from build123d import *

# Parameters (mm, degrees)
BOSS_EXTRUDE1_DEPTH = 10
SKETCH2_W           = 40
SKETCH2_H           = 10
SKETCH2_R           = 1.5
BOSS_EXTRUDE2_DEPTH = 2
FILLET1_R           = 1
SKETCH3_R           = 1.6
CUT_EXTRUDE1_DEPTH  = 35.583232932


with BuildPart() as part:
    # Sketch1 → Boss-Extrude1 (new body)
    with BuildSketch(Plane.XY):
        Polygon((-10, 10), (-10, -10), (-10, -14), (-8, -14), (-8, -8), (-8, 8), (8, 8), (8, -8), (8, -14), (10, -14), (10, -10), (10, 10), align=None)
    extrude(amount=BOSS_EXTRUDE1_DEPTH)

    # Sketch2 → Boss-Extrude2 (add)
    with BuildSketch(Plane(origin=(0, 10, 0), x_dir=(1, 0, 0), z_dir=(0, 1, 0))):
        with Locations((0, -5)):
            Rectangle(SKETCH2_W, SKETCH2_H)
        with Locations(Location((-15, -5, 0), (0, 0, 270))):
            Circle(SKETCH2_R, mode=Mode.SUBTRACT)
        with Locations(Location((15, -5, 0), (0, 0, 90))):
            Circle(SKETCH2_R, mode=Mode.SUBTRACT)
    extrude(amount=BOSS_EXTRUDE2_DEPTH)

    # Fillet1
    fillet1_edges = [part.edges().sort_by_distance(p)[0] for p in [
        (-10, 10, 5),
        (10, 10, 5),
    ]]
    fillet(fillet1_edges, radius=FILLET1_R)

    # Sketch3 → Cut-Extrude1 (cut, through all)
    with BuildSketch(Plane(origin=(10, 0, 0), x_dir=(0, 0, -1), z_dir=(1, 0, 0))):
        with Locations((-5, -9.930512369)):
            Circle(SKETCH3_R)
    extrude(amount=-CUT_EXTRUDE1_DEPTH, mode=Mode.SUBTRACT)


solid = part.part
Geometry: final body of the model. Coordinates: model frame, mm. A direction names the side the tool comes from. Give positions to 0.01 mm unless a question says otherwise; leave off trailing zeros. Order: outer loops, then holes, each group sorted by start corner. A loop starts at its lowest first (then second) coordinate and runs counter-clockwise, first axis right, second up. Notation, with made-up numbers: (57, 58.5) -> (112, 58.5) arc R19 cw to (112, 90.5) -> close; hole circle Ø3 at (88, -6.5). An arc over 180 degrees is marked (long way). Answer as a JSON object with one key per item and string values.
Q1. Section D-D (z = 4.5). State how many separate pieces and enclosed holes the cut face has, plus the area to 3 significant figures.
Entries:
{"separate pieces": "5", "enclosed holes": "0", "area": "185 mm^2"}
Q2. Section B-B (x = -15). Output: boundary loops of the cut face in (y, z).
Entries:
{"outline": "(10, 0) -> (12, 0) -> (12, 3.5) -> (10, 3.5) -> close; (10, 6.5) -> (12, 6.5) -> (12, 10) -> (10, 10) -> close"}
Q3. Material intervals for probe 1 along X at (y, z) = (11.5, 5); probe 2 along X at (y, z) = (-7.75, 9.5); probe 3 along Z at (x, y) = (15, 11.3), sorted ascending.
Entries:
{"probe 1": "x = -20 to -16.5, -13.5 to 13.5, 16.5 to 20", "probe 2": "x = -10 to -8, 8 to 10", "probe 3": "z = 0 to 3.5, 6.5 to 10"}
Q4. Section A-A (y = -6.5). Output: boundary loops of the cut face in (x, z), plus the area to 3 significant figures.
Entries:
{"outline": "(-10, 0) -> (-8, 0) -> (-8, 10) -> (-10, 10) -> close; (8, 0) -> (10, 0) -> (10, 10) -> (8, 10) -> close", "area": "40.0 mm^2"}
Q5. Access query for faces 5 (the flat face through (0, 9, 10)), 6 (the flat face through (16.4, 10, 3.8)), 7 (the flat face through (-8, -3, 5)), 8 (the flat face through (-17, 10, 5)). Directions: +Z, -Z, +X, -X, +Y, -Y. A direction counts if a zero-diameter tool reaches every point of the face in a straight line with its end or side. Return the directions, or none.
Entries:
{"face 5": "+Z, +X, -X, +Y, -Y", "face 6": "+Z, -Z, +X, -Y", "face 7": "+Z, -Z, -Y", "face 8": "+Z, -Z, -X, -Y"}
Q6. Draft query along X for faces 1 (the flat face through (8, -3, 5)), 2 (the flat face through (10, -3, 5)), 3 (the cylindrical face through (14.93, 10.99, 6.5)), 4 (the cylindrical face through (-10.301, 9.715, 5.07)). Return one class per face: released by +X, released by -X, zero draft, split by the parting line, or undercut.
Entries:
{"face 1": "undercut", "face 2": "released by +X", "face 3": "undercut", "face 4": "released by -X"}
Q7. Section C-C (z = 8). Output: boundary loops of the cut face in (x, y), plus the area to 3 significant figures.
Entries:
{"outline": "(-20, 10) -> (-11, 10) arc R1 cw to (-10, 9) -> (-10, -14) -> (-8, -14) -> (-8, 8) -> (8, 8) -> (8, -14) -> (10, -14) -> (10, 9) arc R1 cw to (11, 10) -> (20, 10) -> (20, 12) -> (-20, 12) -> close", "area": "208 mm^2"}
Q8. First-contact query: pin 1 (2.5 mm diameter, centred on x = 14, z = 6.5, fed in from -Y); pin 2 (5 mm diameter, centred on x = -4, z = 5, fed in from -Y); pin 3 (5 mm diameter, centred on y = 0.5, z = 2.5, fed in from -X). Flat tips, straight axial feed; report the tip coordinate or a pass-through.
Entries:
{"pin 1": "stops at y = 10", "pin 2": "stops at y = 8", "pin 3": "stops at x = -10"}
